Could you check a few things on this model? Use its own coordinates, in mm. Give positions to 0.01 mm unless a question says otherwise; leave off trailing zeros. Loops run counter-clockwise (first coordinate to the right, second up) from the corner with the lowest first, then second, coordinate; pieces in that order, holes last. Notation, with made-up numbers: (37.25, 46.5) - (80.25, 46.5) arc R22 cw to (80.25, 64.5) - close; hole circle Ø10 at (84.25, 63). An arc over 180 degrees is marked (long way). Use CSV: the item, a comma, the result in double quotes.
from build123d import *

# Parameters (mm, degrees)
SKETCH1_R           = 7.5
SKETCH1_R_2         = 30
BOSS_EXTRUDE1_DEPTH = 10


with BuildPart() as part:
    # Sketch1 → Boss-Extrude1 (new body)
    with BuildSketch(Plane(origin=(0, 0, 0), x_dir=(1, 0, 0), z_dir=(0, 1, 0))):
        Polygon((287.272653599, -28.421045507), (-119.022979389, 262.995938582), (-168.24967421, -234.574893076), align=None)
        with Locations((-62.5, 138.101451046)):
            Circle(SKETCH1_R, mode=Mode.SUBTRACT)
        with Locations((150.849364905, -14.924137787)):
            Circle(SKETCH1_R, mode=Mode.SUBTRACT)
        with Locations((-88.349364905, -123.17731326)):
            Circle(SKETCH1_R, mode=Mode.SUBTRACT)
        Circle(SKETCH1_R_2, mode=Mode.SUBTRACT)
    extrude(amount=BOSS_EXTRUDE1_DEPTH)


solid = part.part
1) Suppose I cut it at A-A (z = 0). Please give me the cut outline in (x, y), plus the area to 3 significant figures.
Answer below:
outline,"(-145.04, 0) - (-30, 0) - (-30, 10) - (-145.04, 10) - close; (30, 0) - (247.65, 0) - (247.65, 10) - (30, 10) - close"
area,"3,330 mm2"
2) We'd pull the mould along Z, two halves only. Please class faces 1 (the flat face through (56.323, 4.93, 132.941)), 2 (the cylindrical face through (-81.196, 4.93, 120.925)), 3 (the flat face through (6, 0, 38)), 4 (the cylindrical face through (157.777, 4.93, 17.797)): +Z half, -Z half, draft (parallel to the pull), parting line (faces both ways), or undercut.
Answer below:
face 1,"+Z half"
face 2,"undercut"
face 3,"draft"
face 4,"undercut"
3) Suppose I cut it at B-B (x = 0). Please give me the cut outline in (y, z), plus the area to 3 significant figures.
Answer below:
outline,"(0, -177.63) - (10, -177.63) - (10, -30) - (0, -30) - close; (0, 30) - (10, 30) - (10, 158.43) - (0, 158.43) - close"
area,"2,760 mm2"
4) Suppose I cut it at C-C (y = 4.25). Please give me the cut outline in (x, z).
Answer below:
outline,"(-168.25, 234.57) - (-119.02, -263) - (287.27, 28.42) - close; hole circle Ø15 at (-88.35, 123.18); hole circle Ø15 at (-62.5, -138.1); hole circle Ø60 at (0, 0); hole circle Ø15 at (150.85, 14.92)"
5) Suppose I cut it at D-D (x = 69.5). Please give me the cut outline in (y, z).
Answer below:
outline,"(0, -127.78) - (10, -127.78) - (10, 126.98) - (0, 126.98) - close"
6) I'm going to push a flat-ended pin straight in: P1, Ø1.5, axis at y = 8, z = 76.5, coming from the -X side. Where does the tip first touch, or does it pass through?
Answer below:
P1,"stops at x = -152.68"
7) I need wall thicknesses on line 1 along Z through (x, y) = (-25.5, 2.5); line 2 along Z through (x, y) = (-90, 1); line 3 along X through (y, z) = (3.75, -20). Which ranges of each line are inside material? Lowest first, please.
Answer below:
line 1,"z = -195.92 to -15.8, 15.8 to 169.97"
line 2,"z = -242.18 to 115.86, 130.49 to 199.16"
line 3,"x = -143.06 to -22.36, 22.36 to 219.76"
